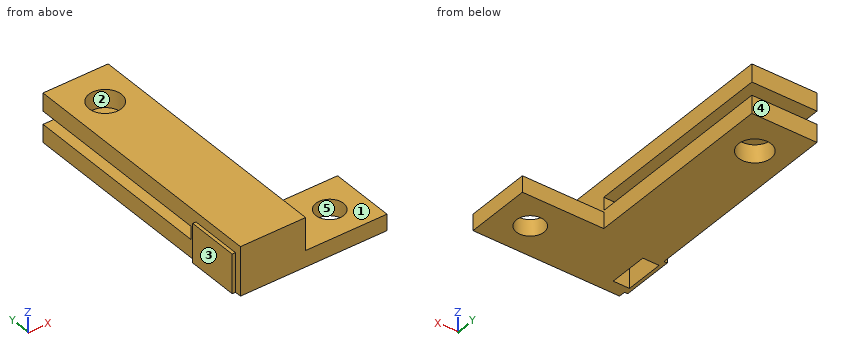
from build123d import *

# Parameters (mm, degrees)
SKETCH1_W           = 20
SKETCH1_H           = 70
BOSS_EXTRUDE1_DEPTH = 15
SKETCH2_W           = 20
SKETCH2_H           = 4
CUT_EXTRUDE1_DEPTH  = 60
SKETCH3_R           = 5
CUT_EXTRUDE2_DEPTH  = 15
SKETCH4_W           = 45
SKETCH4_H           = 20
BOSS_EXTRUDE2_DEPTH = 5
SKETCH7_R           = 4.25
CUT_EXTRUDE4_DEPTH  = 8
SKETCH8_W           = 20
SKETCH8_H           = 10
BOSS_EXTRUDE3_DEPTH = 10
SKETCH9_W           = 5
SKETCH9_H           = 12
CUT_EXTRUDE5_DEPTH  = 10
SKETCH10_W          = 12
SKETCH10_H          = 16
BOSS_EXTRUDE4_DEPTH = 1


with BuildPart() as part:
    # Sketch1 → Boss-Extrude1 (new body)
    with BuildSketch(Plane.XY):
        with Locations((0, -4.140597693)):
            Rectangle(SKETCH1_W, SKETCH1_H)
    extrude(amount=BOSS_EXTRUDE1_DEPTH)

    # Sketch2 → Cut-Extrude1 (cut)
    with BuildSketch(Plane(origin=(0, 30.859402307, 0), x_dir=(1, 0, 0), z_dir=(0, 1, 0))):
        with Locations((0, -7.5)):
            Rectangle(SKETCH2_W, SKETCH2_H)
    extrude(amount=-CUT_EXTRUDE1_DEPTH, mode=Mode.SUBTRACT)

    # Sketch3 → Cut-Extrude2 (cut)
    with BuildSketch(Plane.XY.offset(15)):
        with Locations((0, 18.859402307)):
            Circle(SKETCH3_R)
    extrude(amount=-CUT_EXTRUDE2_DEPTH, mode=Mode.SUBTRACT)

    # Sketch4 → Boss-Extrude2 (add)
    with BuildSketch(Plane(origin=(0, 0, 0), x_dir=(-1, 0, 0), z_dir=(0, 0, -1))):
        with Locations((-12.5, -39.140597693)):
            Rectangle(SKETCH4_W, SKETCH4_H)
    extrude(amount=-BOSS_EXTRUDE2_DEPTH)

    # Sketch7 → Cut-Extrude4 (cut)
    with BuildSketch(Plane(origin=(0, 0, 0), x_dir=(-1, 0, 0), z_dir=(0, 0, -1))):
        with Locations((-25, -39.122753145)):
            Circle(SKETCH7_R)
    extrude(amount=-CUT_EXTRUDE4_DEPTH, mode=Mode.SUBTRACT)

    # Sketch8 → Boss-Extrude3 (add)
    with BuildSketch(Plane.XY.offset(5)):
        with Locations((0, -44.140597693)):
            Rectangle(SKETCH8_W, SKETCH8_H)
    extrude(amount=BOSS_EXTRUDE3_DEPTH)

    # Sketch9 → Cut-Extrude5 (cut)
    with BuildSketch(Plane(origin=(0, 0, 0), x_dir=(-1, 0, 0), z_dir=(0, 0, -1))):
        with Locations((7.5, -39.122753145)):
            Rectangle(SKETCH9_W, SKETCH9_H)
    extrude(amount=-CUT_EXTRUDE5_DEPTH, mode=Mode.SUBTRACT)

    # Sketch10 → Boss-Extrude4 (add)
    with BuildSketch(Plane.ZY.offset(10)):
        with Locations((6, -39.122753145)):
            Rectangle(SKETCH10_W, SKETCH10_H)
    extrude(amount=BOSS_EXTRUDE4_DEPTH)


solid = part.part
Part model, mm, in its own coordinate system. Face numbers are marked on the shaded views. A direction names the side the tool comes from. Coordinates: 2 decimals unless noted, no trailing zeros. Loops run counter-clockwise (first coordinate to the right, second up) from the corner with the lowest first, then second, coordinate; pieces in that order, holes last. Notation, with made-up numbers: (46, 71) - (100, 71) arc R8 cw to (100, 75) - close; hole circle Ø5 at (16, 73). An arc over 180 degrees is marked (long way). Write each question's results on one line, items separated by ' | '. Start each with the question number.
Q1. Slice it at A-A on y = -20. Give the cut face in (x, z).
Q2. Slice it at B-B on z = 7.25. Give the cut face in (x, y), and give its area (3 significant figures).
Q3. Which spindle directions (+Z, -Z, +X, -X, +Y, -Y) get a long thin tool onto all of the face, cutting with end or side? Do the marked faces 1 and 2. Say none if no direction does.
Q4. Slice it at C-C on x = 25. Give the cut face in (y, z), and give its area (3 significant figures).
Q5. Drop flat-ended pins along their axis: pin 1 Ø8 at (y, z) = (-1, 6.5) entering from +X; pin 2 Ø1 at (x, z) = (22.5, 5) entering from +Y; pin 3 Ø1.5 at (x, z) = (5.5, 9) entering from +Y; pin 4 Ø7.5 at (y, z) = (-16.5, 6) entering from -X. Give the stop position or say it passes through.
Q6. Probe line 1 along Z through (x, y) = (-5, -21.5); line 2 along Y through (x, z) = (25, 3.75); line 3 along Y through (x, z) = (0, 11.45). List the from-to ranges inside material, lowest first.
Q7. Slice it at D-D on x = 0. Give the cut face in (y, z), and give its area (3 significant figures).
Q8. Two-plate mould, pull along X, no slides. Class the marked faces 3, 4 and 5: +X half, -X half, draft (parallel to the pull), parting line (faces both ways), or undercut.
Answer:
1) outline: (-10, 0) - (10, 0) - (10, 5.5) - (-10, 5.5) - close; (-10, 9.5) - (10, 9.5) - (10, 15) - (-10, 15) - close
2) outline: (-11, -47.12) - (-10, -47.12) - (-10, -49.14) - (10, -49.14) - (10, -29.14) - (-10, -29.14) - (-10, -31.12) - (-11, -31.12) - close; hole (-10, -45.12) - (-5, -45.12) - (-5, -33.12) - (-10, -33.12) - close | area: 356 mm2
3) face 1: +Z, +X, +Y, -Y | face 2: +Z, -Z
4) outline: (-49.14, 0) - (-43.37, 0) - (-43.37, 5) - (-49.14, 5) - close; (-34.87, 0) - (-29.14, 0) - (-29.14, 5) - (-34.87, 5) - close | area: 57.5 mm2
5) pin 1: stops at x = 10 | pin 2: stops at y = -29.14 | pin 3: stops at y = 30.86 | pin 4: stops at x = -10
6) line 1: z = 0 to 5.5, 9.5 to 15 | line 2: y = -49.14 to -43.37, -34.87 to -29.14 | line 3: y = -49.14 to 13.86, 23.86 to 30.86
7) outline: (-49.14, 0) - (13.86, 0) - (13.86, 5.5) - (-29.14, 5.5) - (-29.14, 9.5) - (13.86, 9.5) - (13.86, 15) - (-49.14, 15) - close; (23.86, 0) - (30.86, 0) - (30.86, 5.5) - (23.86, 5.5) - close; (23.86, 9.5) - (30.86, 9.5) - (30.86, 15) - (23.86, 15) - close | area: 850 mm2
8) face 3: -X half | face 4: draft | face 5: undercut
